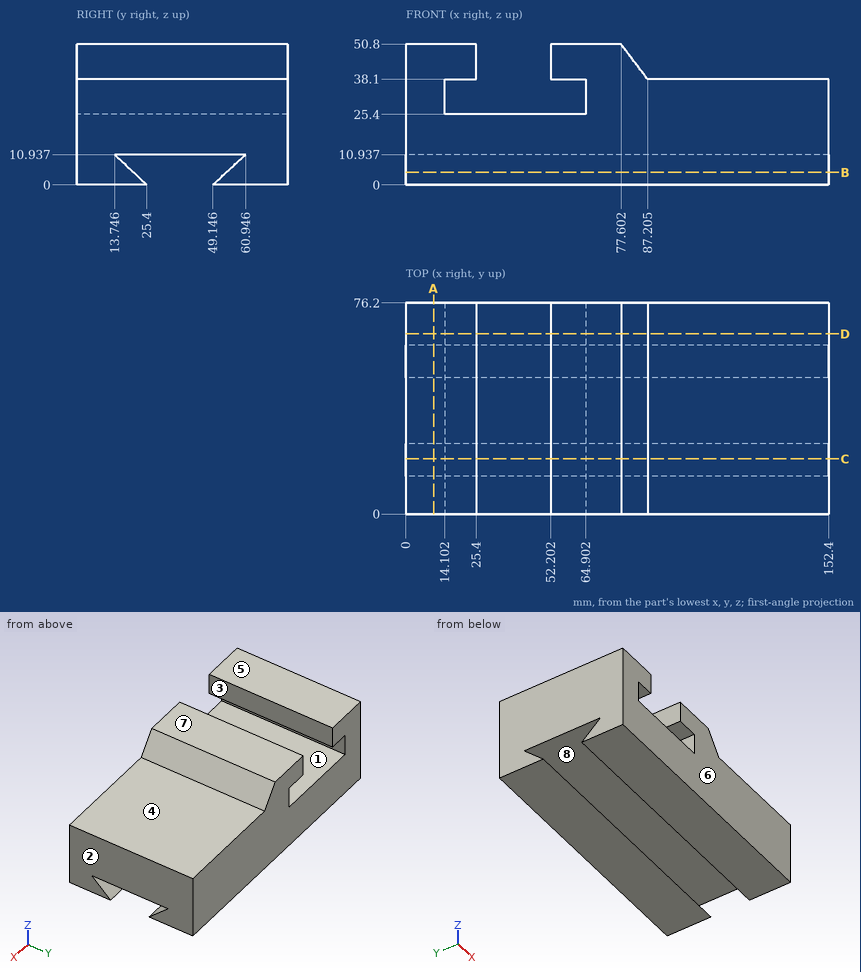
Input: dimensioned drawing with shaded views. Units: mm. Origin: part minimum x, y, z. A direction names the side the tool comes from. Round coordinates to 2 decimals unless told otherwise and drop trailing zeros. Loops run counter-clockwise (first coordinate to the right, second up) from the corner with the lowest first, then second, coordinate; pieces in that order, holes last. Notation, with made-up numbers: M 52.25,2.25 L 67.25,2.25 A29 cw 67.25,40.25 Z; hole C 67,53.5 d4. An arc over 180 degrees is marked long. Answer in a Markdown table with one row per item. Add a question column.
1. Section B-B (z = 4.5). Output: boundary loops of the cut face in (x, y) (1 decimal).
2. Section C-C (y = 20). Output: boundary loops of the cut face in (x, z) (1 decimal).
3. Section D-D (y = 65). Output: boundary loops of the cut face in (x, z) (1 decimal), and give its area (3 significant figures).
4. Ray query, probe 1 along X at (y, z) = (4, 32.5); probe 2 along Z at (x, y) = (19, 67.5); probe 3 along Z at (x, y) = (143.5, 29). Return the intervals inside material, ascending.
5. Contact query for flat-ended pins moving along their axis: pin 1 (9 mm diameter, centred on x = 20.5, y = 55, fed in from -Z); pin 2 (19.5 mm diameter, centred on x = 118.5, y = 28, fed in from +Z). Output: stop coordinate, or through.
6. Mould query, pull axis Y, two halves, no side actions, for the marked faces 6, 7 and 8. Classes: released by +Y, released by -Y, zero draft, split by the parting line, or undercut.
7. Set-up query: the marked faces 1, 2, 3, 4 and 5. Return all of +Z, -Z, +X, -X, +Y, -Y with unobstructed straight access to the full face (end or side cutting, diameter ignored); none if empty.
8. Section A-A (x = 10). Output: boundary loops of the cut face in (y, z).
Values follow:
| question | item | result |
|---|---|---|
| 1 | outline | M 0,0 L 152.4,0 L 152.4,20.6 L 0,20.6 Z; M 0,54 L 152.4,54 L 152.4,76.2 L 0,76.2 Z |
| 2 | outline | M 0,0 L 152.4,0 L 152.4,5.1 L 0,5.1 Z; M 0,10.9 L 152.4,10.9 L 152.4,38.1 L 87.2,38.1 L 77.6,50.8 L 52.2,50.8 L 52.2,38.1 L 64.9,38.1 L 64.9,25.4 L 14.1,25.4 L 14.1,38.1 L 25.4,38.1 L 25.4,50.8 L 0,50.8 Z |
| 3 | outline | M 0,0 L 152.4,0 L 152.4,38.1 L 87.2,38.1 L 77.6,50.8 L 52.2,50.8 L 52.2,38.1 L 64.9,38.1 L 64.9,25.4 L 14.1,25.4 L 14.1,38.1 L 25.4,38.1 L 25.4,50.8 L 0,50.8 Z |
| 3 | area | 5,870 mm^2 |
| 4 | probe 1 | 0 to 14.1, 64.9 to 152.4 |
| 4 | probe 2 | 0 to 25.4, 38.1 to 50.8 |
| 4 | probe 3 | 10.94 to 38.1 |
| 5 | pin 1 | z = 0 |
| 5 | pin 2 | z = 38.1 |
| 6 | face 6 | released by -Y |
| 6 | face 7 | zero draft |
| 6 | face 8 | undercut |
| 7 | face 1 | +Y, -Y |
| 7 | face 2 | +Z, -Z, +X, +Y, -Y |
| 7 | face 3 | +Z, +Y, -Y |
| 7 | face 4 | +Z, +X, +Y, -Y |
| 7 | face 5 | +Z, +X, -X, +Y, -Y |
| 8 | outline | M 0,0 L 25.4,0 L 13.75,10.94 L 60.95,10.94 L 49.15,0 L 76.2,0 L 76.2,50.8 L 0,50.8 Z |
